Read the model definition and answer for the solid it produces. Units are mm, in the model's axes. Face numbers are marked on the shaded views. A direction names the side the tool comes from. Coordinates: 2 decimals unless noted, no trailing zeros. Loops run counter-clockwise (first coordinate to the right, second up) from the corner with the lowest first, then second, coordinate; pieces in that order, holes last. Notation, with made-up numbers: (35, 73.25) - (87, 73.25) arc R23 ccw to (87, 92.25) - close; hole circle Ø6 at (63.25, 84). An arc over 180 degrees is marked (long way). One line per item, written item: value. Start each with the question number.
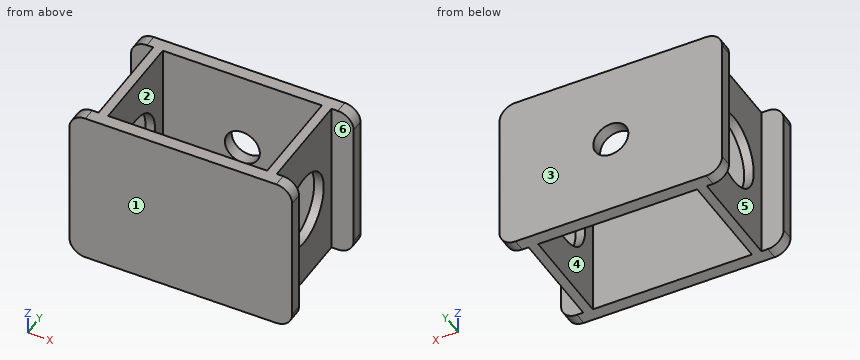
from build123d import *

# Parameters (mm, degrees)
BOSS_EXTRUDE1_DEPTH = 4
SKETCH2_W           = 3
SKETCH2_H           = 50
BOSS_EXTRUDE4_DEPTH = 32
SKETCH4_W           = 50
SKETCH4_H           = 50
SKETCH4_W_2         = 3
BOSS_EXTRUDE5_DEPTH = 4
SKETCH6_R           = 11.5
CUT_EXTRUDE1_DEPTH  = 106
SKETCH7_R           = 5.5
CUT_EXTRUDE2_DEPTH  = 10


with BuildPart() as part:
    # Sketch1 → Boss-Extrude1 (new body)
    with BuildSketch(Plane(origin=(0, 0, 0), x_dir=(1, 0, 0), z_dir=(0, 1, 0))):
        with BuildLine():
            Line((-30, 25), (30, 25))
            ThreePointArc((30, 25), (33.535533906, 23.535533906), (35, 20))
            Line((35, 20), (35, -20))
            ThreePointArc((35, -20), (33.535533906, -23.535533906), (30, -25))
            Line((30, -25), (-30, -25))
            ThreePointArc((-30, -25), (-33.535533906, -23.535533906), (-35, -20))
            Line((-35, -20), (-35, 20))
            ThreePointArc((-35, 20), (-33.535533906, 23.535533906), (-30, 25))
        make_face()
    extrude(amount=BOSS_EXTRUDE1_DEPTH)

    # Sketch2 → Boss-Extrude4 (add)
    with BuildSketch(Plane(origin=(0, 4, 0), x_dir=(1, 0, 0), z_dir=(0, 1, 0))):
        with Locations((-26.5, 0)):
            Rectangle(SKETCH2_W, SKETCH2_H)
        with Locations((26.5, 0)):
            Rectangle(SKETCH2_W, SKETCH2_H)
    extrude(amount=BOSS_EXTRUDE4_DEPTH)

    # Sketch4 → Boss-Extrude5 (add)
    with BuildSketch(Plane(origin=(0, 36, 0), x_dir=(1, 0, 0), z_dir=(0, 1, 0))):
        Rectangle(SKETCH4_W, SKETCH4_H)
        with BuildLine():
            Line((-35, 20), (-35, -20))
            ThreePointArc((-35, -20), (-33.535533906, -23.535533906), (-30, -25))
            Line((-30, -25), (-28, -25))
            Line((-28, -25), (-28, 25))
            Line((-28, 25), (-30, 25))
            ThreePointArc((-30, 25), (-33.535533906, 23.535533906), (-35, 20))
        make_face()
        with BuildLine():
            Line((35, -20), (35, 20))
            ThreePointArc((35, 20), (33.535533906, 23.535533906), (30, 25))
            Line((30, 25), (28, 25))
            Line((28, 25), (28, -25))
            Line((28, -25), (30, -25))
            ThreePointArc((30, -25), (33.535533906, -23.535533906), (35, -20))
        make_face()
        with Locations((26.5, 0)):
            Rectangle(SKETCH4_W_2, SKETCH4_H)
        with Locations((-26.5, 0)):
            Rectangle(SKETCH4_W_2, SKETCH4_H)
    extrude(amount=BOSS_EXTRUDE5_DEPTH)

    # Sketch6 → Cut-Extrude1 (cut)
    with BuildSketch(Plane(origin=(28, 0, 0), x_dir=(0, 0, -1), z_dir=(1, 0, 0))):
        with Locations((0, 20)):
            Circle(SKETCH6_R)
    extrude(amount=-CUT_EXTRUDE1_DEPTH, mode=Mode.SUBTRACT)

    # Sketch7 → Cut-Extrude2 (cut)
    with BuildSketch(Plane(origin=(0, 40, 0), x_dir=(1, 0, 0), z_dir=(0, 1, 0))):
        Circle(SKETCH7_R)
    extrude(amount=-CUT_EXTRUDE2_DEPTH, mode=Mode.SUBTRACT)


solid = part.part
1) Section D-D, the plane y = 34.5 is taken. Determine the outline of the cut face in (x, z), and give its area (3 significant figures).
2) Section A-A, the plane y = 20 is taken. Determine the outline of the cut face in (x, z), and give its area (3 significant figures).
3) Section B-B, the plane z = 0 is taken. Determine the outline of the cut face in (x, y).
4) For the marked faces 4, 5 and 6, determine the directions among +Z, -Z, +X, -X, +Y, -Y from which every point of the face is accessible in a straight line to the end or side of a thin tool.
5) Straight lines are drawn through the part: L1, parallel to X at y = 9, z = 5; L2, parallel to Y at x = -18, z = -10; L3, parallel to X at y = 39, z = 0. For each, find the intervals that lie inside material, in ascending order.
6) Flat-ended cylindrical pins translate along their axes: P1, Ø16, axis at y = 17.5, z = 3, coming from the -X side; P2, Ø1.5, axis at y = 20.5, z = 16.5, coming from the +X side. Find the tip coordinate at first contact, or state that the pin passes through.
7) Determine the mould class of the marked faces 1, 2 and 3 for opening direction Y: released by +Y, released by -Y, zero draft, split by the parting line, or undercut.
8) Section C-C, the plane x = -7 is taken. Determine the outline of the cut face in (y, z), and give its area (3 significant figures).
Answer below:
1. outline: (-28, -25) - (-25, -25) - (-25, 25) - (-28, 25) - close; (25, -25) - (28, -25) - (28, 25) - (25, 25) - close
1. area: 300 mm2
2. outline: (-28, -25) - (-25, -25) - (-25, -11.5) - (-28, -11.5) - close; (-28, 11.5) - (-25, 11.5) - (-25, 25) - (-28, 25) - close; (25, -25) - (28, -25) - (28, -11.5) - (25, -11.5) - close; (25, 11.5) - (28, 11.5) - (28, 25) - (25, 25) - close
2. area: 162 mm2
3. outline: (-35, 0) - (35, 0) - (35, 4) - (28, 4) - (28, 8.5) - (25, 8.5) - (25, 4) - (-25, 4) - (-25, 8.5) - (-28, 8.5) - (-28, 4) - (-35, 4) - close; (-35, 36) - (-28, 36) - (-28, 31.5) - (-25, 31.5) - (-25, 36) - (-5.5, 36) - (-5.5, 40) - (-35, 40) - close; (5.5, 36) - (25, 36) - (25, 31.5) - (28, 31.5) - (28, 36) - (35, 36) - (35, 40) - (5.5, 40) - close
4. face 4: +Z, -Z
4. face 5: +Z, -Z, -X
4. face 6: +Z, -Z, +X
5. L1: -28 to -25, 25 to 28
5. L2: 0 to 4, 36 to 40
5. L3: -35 to -5.5, 5.5 to 35
6. P1: x = -28
6. P2: x = 28
7. face 1: released by -Y
7. face 2: undercut
7. face 3: released by +Y
8. outline: (0, -25) - (4, -25) - (4, 25) - (0, 25) - close; (36, -25) - (40, -25) - (40, 25) - (36, 25) - close
8. area: 400 mm2
